Design review of the part built by this model. Coordinates are the model's own, in mm. A direction names the side the tool comes from. Coordinates: 2 decimals unless noted, no trailing zeros. Loops run counter-clockwise (first coordinate to the right, second up) from the corner with the lowest first, then second, coordinate; pieces in that order, holes last. Notation, with made-up numbers: (-19, 35) -> (26, 35) arc R15 cw to (26, 42) -> close; hole circle Ø10 at (-7, 45). An arc over 180 degrees is marked (long way). One line per item, written item: value. Start each with the question number.
1. For probe 1 along Y at (x, z) = (10.75, 0); probe 2 along Z at (x, y) = (-0.75, -16); probe 3 along Y at (x, z) = (-8.75, -12.5), list the stretches that pass through material, from the lowest coordinate up.
2. Add section A-A on x = -6.25. Write out the cut boundary in (y, z), plus the area to 3 significant figures.
3. Draft analysis for pull direction X (two halves, no side actions). For faces 5 (the flat face through (12.5, 26.5, 30.2)), 6 (the flat face through (-10, 4, 0)), 7 (the flat face through (-5, -6, 14)), 8 (the flat face through (-12.5, 26.5, -30.2)), state which applies: pulls with the +X half, pulls with the -X half, needs draft (parallel to the pull), parting line crosses it, or undercut.
4. Add section D-D on y = -23. Write out the cut boundary in (x, z), plus the area to 3 significant figures.
5. Add section C-C on z = 37. Write out the cut boundary in (x, y), plus the area to 3 significant figures.
6. Insertion check: pin 1 (1.5 mm diameter, centred on x = -4.5, y = 8.5, fed in from -Z); pin 2 (9 mm diameter, centred on y = 14.03, z = 17.59, fed in from -X); pin 3 (10 mm diameter, centred on x = 12, y = 32, fed in from -Z); pin 4 (1.5 mm diameter, centred on y = 13, z = -12, fed in from -X). Each pin has a flat end and moves straight along its axis. Give the tip position at first contact, or say it passes through.
7. Machinability: for faces 1 (the cylindrical face through (-0.18, -39.05, 8.67)), 2 (the cylindrical face through (-0.07, 17.62, 1.08)), 3 (the flat face through (2, 11, 4)), 4 (the cylindrical face through (-10.07, 0.66, 14.985)), which of the approach directions +Z, -Z, +X, -X, +Y, -Y give a long, thin tool a straight path to every point of the face, cutting with its end or side? Answer none if there is none.
8. Add section B-B on y = 22.5. Write out the cut boundary in (x, z).
```python
from build123d import *

# Parameters (mm, degrees)
BOSS_EXTRUDE1_DEPTH      = 15
BOSS_EXTRUDE1_DEPTH_BACK = 15
SKETCH1_R                = 15
SKETCH2_R                = 13
SKETCH2_R_2              = 3.5
BOSS_EXTRUDE2_DEPTH      = 5
BOSS_EXTRUDE3_DEPTH      = 5
BOSS_EXTRUDE3_DEPTH_BACK = 5
SKETCH3_R                = 30
SKETCH3_R_2              = 5
SKETCH3_R_3              = 13.5
BOSS_EXTRUDE4_DEPTH      = 15
BOSS_EXTRUDE4_DEPTH_BACK = 15
SKETCH4_R                = 40
SKETCH4_R_2              = 30


with BuildPart() as part:
    # Sketch1 → Boss-Extrude1 (new, two sides: drawn at the far end of the back side and taken through both)
    with BuildSketch(Plane(origin=(0, 0, 0), x_dir=(0, 0, -1), z_dir=(1, 0, 0)).offset(-BOSS_EXTRUDE1_DEPTH_BACK)):
        Circle(SKETCH1_R)
        with BuildLine():
            Line((-4, 9.16515139), (-4, 12))
            Line((-4, 12), (4, 12))
            Line((4, 12), (4, 9.16515139))
            ThreePointArc((4, 9.16515139), (0, -10), (-4, 9.16515139))
        make_face(mode=Mode.SUBTRACT)
    extrude(amount=BOSS_EXTRUDE1_DEPTH + BOSS_EXTRUDE1_DEPTH_BACK)

    # Sketch2 → Boss-Extrude2 (add)
    with BuildSketch(Plane.ZY.offset(15)):
        Circle(SKETCH2_R)
        Circle(SKETCH2_R_2, mode=Mode.SUBTRACT)
    extrude(amount=-BOSS_EXTRUDE2_DEPTH)

    # Sketch3 → Boss-Extrude3 (add, two sides: drawn at the far end of the back side and taken through both)
    with BuildSketch(Plane(origin=(0, 0, 0), x_dir=(0, 0, -1), z_dir=(1, 0, 0)).offset(-BOSS_EXTRUDE3_DEPTH_BACK)):
        Circle(SKETCH3_R)
        with Locations((0, 22.5)):
            Circle(SKETCH3_R_2, mode=Mode.SUBTRACT)
        with Locations((17.591208356, 14.028520542)):
            Circle(SKETCH3_R_2, mode=Mode.SUBTRACT)
        with Locations((21.935878024, -5.006721014)):
            Circle(SKETCH3_R_2, mode=Mode.SUBTRACT)
        with Locations((9.76238413, -20.271799528)):
            Circle(SKETCH3_R_2, mode=Mode.SUBTRACT)
        with Locations((-9.76238413, -20.271799528)):
            Circle(SKETCH3_R_2, mode=Mode.SUBTRACT)
        with Locations((-21.935878024, -5.006721014)):
            Circle(SKETCH3_R_2, mode=Mode.SUBTRACT)
        with Locations((-17.591208356, 14.028520542)):
            Circle(SKETCH3_R_2, mode=Mode.SUBTRACT)
        Circle(SKETCH3_R_3, mode=Mode.SUBTRACT)
    extrude(amount=BOSS_EXTRUDE3_DEPTH + BOSS_EXTRUDE3_DEPTH_BACK)

    # Sketch4 → Boss-Extrude4 (add, two sides: drawn at the far end of the back side and taken through both)
    with BuildSketch(Plane(origin=(0, 0, 0), x_dir=(0, 0, -1), z_dir=(1, 0, 0)).offset(-BOSS_EXTRUDE4_DEPTH_BACK)):
        Circle(SKETCH4_R)
        Circle(SKETCH4_R_2, mode=Mode.SUBTRACT)
    extrude(amount=BOSS_EXTRUDE4_DEPTH + BOSS_EXTRUDE4_DEPTH_BACK)

    # Sketch5 → Revolve1 (revolve)
    with BuildSketch(Plane.XY, mode=Mode.PRIVATE) as revolve1_sk:
        Polygon((-15, 36), (-15, 45), (-12.5, 45), (-12.5, 37), (12.5, 37), (12.5, 45), (15, 45), (15, 36), align=None)
    revolve(revolve1_sk.sketch.rotate(Axis((0, 0, 0), (1, 0, 0)), 90), axis=Axis((0, 0, 0), (1, 0, 0)))


solid = part.part
```
Worked answers:
1. probe 1: y = -40 to -30, -15 to -10, 12 to 15, 30 to 40
1. probe 2: z = -36.66 to -12.36, -7.16 to 7.16, 12.36 to 36.66
1. probe 3: y = -38 to -27.27, -8.29 to 8.29, 27.27 to 38
2. outline: circle Ø80 at (0, 0); circle Ø30 at (0, 0); hole circle Ø60 at (0, 0); hole (9.17, -4) -> (12, -4) -> (12, 4) -> (9.17, 4) arc R10 ccw (long way) to start
2. area: 2,570 mm²
3. face 5: undercut
3. face 6: pulls with the +X half
3. face 7: pulls with the -X half
3. face 8: undercut
4. outline: (-15, -38.68) -> (-12.5, -38.68) -> (-12.5, -32.73) -> (12.5, -32.73) -> (12.5, -38.68) -> (15, -38.68) -> (15, -19.26) -> (5, -19.26) -> (5, -13.95) -> (-5, -13.95) -> (-5, -19.26) -> (-15, -19.26) -> close; (-15, 19.26) -> (-5, 19.26) -> (-5, 13.95) -> (5, 13.95) -> (5, 19.26) -> (15, 19.26) -> (15, 38.68) -> (12.5, 38.68) -> (12.5, 32.73) -> (-12.5, 32.73) -> (-12.5, 38.68) -> (-15, 38.68) -> close; (-5, -5.57) -> (5, -5.57) -> (5, 5.57) -> (-5, 5.57) -> close
4. area: 1,090 mm²
5. outline: (-15, -25.61) -> (-12.5, -25.61) -> (-12.5, -15.2) -> (12.5, -15.2) -> (12.5, -25.61) -> (15, -25.61) -> (15, 25.61) -> (12.5, 25.61) -> (12.5, 15.2) -> (-12.5, 15.2) -> (-12.5, 25.61) -> (-15, 25.61) -> close
5. area: 1,020 mm²
6. pin 1: stops at z = -39.24
6. pin 2: passes through
6. pin 3: stops at z = -35.98
6. pin 4: stops at x = -5
7. face 1: none
7. face 2: +X, -X
7. face 3: +X
7. face 4: -X
8. outline: (-15, -38.97) -> (-12.5, -38.97) -> (-12.5, -33.07) -> (12.5, -33.07) -> (12.5, -38.97) -> (15, -38.97) -> (15, -19.84) -> (5, -19.84) -> (5, -5) -> (-5, -5) -> (-5, -19.84) -> (-15, -19.84) -> close; (-15, 19.84) -> (-5, 19.84) -> (-5, 5) -> (5, 5) -> (5, 19.84) -> (15, 19.84) -> (15, 38.97) -> (12.5, 38.97) -> (12.5, 33.07) -> (-12.5, 33.07) -> (-12.5, 38.97) -> (-15, 38.97) -> close
